```python
from build123d import *

# Parameters (mm, degrees)
F3_W      = 508
F3_H      = 508
F4_DEPTH  = 50.8
F5_W      = 406.4
F5_H      = 101.6
F6_DEPTH  = 406.4
F8_DEPTH  = 304.801
F9_SIZE   = 99.06
F10_SIZE  = 99.06
F15_R     = 0.127
F16_DEPTH = 304.801


with BuildPart() as f4:
    # F3 (on Top) → F4 (new body)
    with BuildSketch(Plane.XY):
        Rectangle(F3_W, F3_H)
    extrude(amount=F4_DEPTH)

    # F5 (on face) → F6 (join)
    with BuildSketch(Plane.XY.offset(50.8)):
        Rectangle(F5_W, F5_H)
    extrude(amount=F6_DEPTH)

    # F7 (on face) → F8 (cut, through all)
    with BuildSketch(Plane.XZ.offset(50.8)):
        Polygon((203.2, 322.3866591478), (203.2, 457.2), (68.3866591478, 457.2), align=None)
        Polygon((-68.3866591478, 457.2), (-203.2, 457.2), (-203.2, 322.3866591478), align=None)
    extrude(amount=-F8_DEPTH, mode=Mode.SUBTRACT)

    # F9
    f9_edges = [f4.edges().sort_by_distance(p)[0] for p in [
        (0, 50.8, 457.2),
    ]]
    chamfer(f9_edges, length=F9_SIZE)

    # F10
    f10_edges = [f4.edges().sort_by_distance(p)[0] for p in [
        (185.32333, 50.8, 340.26333),
        (-185.32333, 50.8, 340.26333),
    ]]
    chamfer(f10_edges, length=F10_SIZE)


with BuildPart() as f4_1:
    # F11: moved
    add(f4.part)


with BuildPart() as f4_2:
    # F14: moved
    add(f4_1.part)

    # F15 (on face) → F16 (cut, through all)
    with BuildSketch(Plane.XZ.offset(50.8)):
        with Locations((0, 292.1)):
            Circle(F15_R)
    extrude(amount=-F16_DEPTH, mode=Mode.SUBTRACT)


solid = f4_2.part
```
For this review, take the finished solid that the model builds, in its own axes (mm). A direction names the side the tool comes from. Coordinates: 2 decimals unless noted, no trailing zeros. Order: outer loops, then holes, each group sorted by start corner. A loop starts at its lowest first (then second) coordinate and runs counter-clockwise, first axis right, second up. Notation, with made-up numbers: (75.5, -31) -> (98.5, -31) arc R3 cw to (98.5, -26) -> close; hole circle Ø10 at (82, 24.25). An arc over 180 degrees is marked (long way). Answer as CSV lines item,"result".
Q1. Clearance check with flat-ended pins moving along their axes: pin 1 Ø1 at (x, z) = (-43.5, 327) entering from -Y; pin 2 Ø12 at (y, z) = (5.5, 104.5) entering from -X; pin 3 Ø2 at (x, y) = (1, -89.5) entering from +Z. State where each tip first meets the part, or that it passes through.
Model answer:
pin 1,"stops at y = -50.8"
pin 2,"stops at x = -203.2"
pin 3,"stops at z = 50.8"
Q2. For faces 1 (the face through (203.2, -1, 155)), 2 (the face through (-203.2, -1, 155)), 3 (the face through (-3, 50.8, 168)), 4 (the face through (-3, -50.8, 251)), list the 3-axis set-ups (+Z, -Z, +X, -X, +Y, -Y) from which the entire face can be reached by the end or side of a thin tool; tool diameter is ignored.
Model answer:
face 1,"+Z, +X, +Y, -Y"
face 2,"+Z, -X, +Y, -Y"
face 3,"+Z, +X, -X, +Y"
face 4,"+Z, +X, -X, -Y"
Q3. Wall thickness on line 1 along Y through (x, z) = (33, 59); line 2 along X through (y, z) = (-2.5, 292.1); line 3 along Z through (x, y) = (115.5, 171.5): over which ranges is each line inside the solid? List them lowest first. Write a range as [from, to].
Model answer:
line 1,"y = [-50.8, 50.8]"
line 2,"x = [-168.77, -0.13], [0.13, 168.77]"
line 3,"z = [0, 50.8]"
Q4. We need section B-B (x = 114.5). State the section outline as (y, z) points.
Model answer:
outline,"(-254, 0) -> (254, 0) -> (254, 50.8) -> (50.8, 50.8) -> (50.8, 270.99) -> (-48.26, 411.09) -> (-50.8, 411.09) -> (-50.8, 50.8) -> (-254, 50.8) -> close"
Q5. We need section C-C (y = 128.5). State the section outline as (x, z) points, plus the area to 3 significant figures.
Model answer:
outline,"(-254, 0) -> (254, 0) -> (254, 50.8) -> (-254, 50.8) -> close"
area,"25,800 mm2"
Q6. We need section D-D (z = 285). State the section outline as (x, y) points.
Model answer:
outline,"(-203.2, -50.8) -> (203.2, -50.8) -> (203.2, -21.82) -> (100.49, 50.8) -> (-100.49, 50.8) -> (-203.2, -21.82) -> close"
